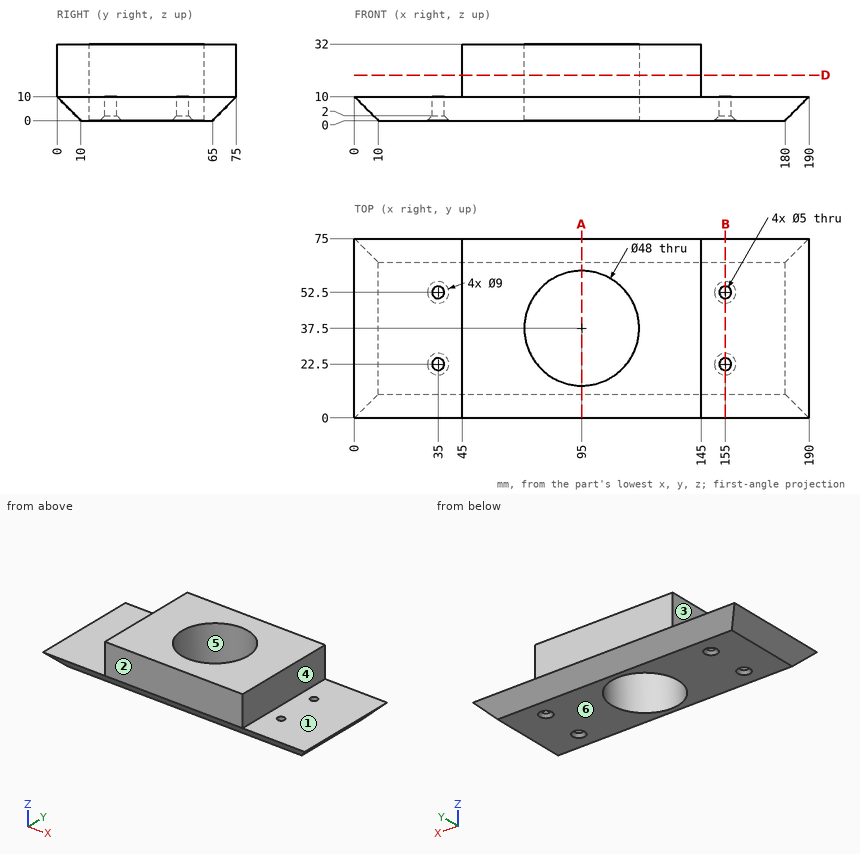
Could you check a few things on this drawing? It's one solid part, dimensions in mm from its lowest x, y, z. A direction names the side the tool comes from. Give positions to 0.01 mm unless a question says otherwise; leave off trailing zeros. Order: outer loops, then holes, each group sorted by start corner. A loop starts at its lowest first (then second) coordinate and runs counter-clockwise, first axis right, second up. Notation, with made-up numbers: (1, 31.5) - (5, 31.5) arc R19 cw to (5, 66.5) - close; hole circle Ø5 at (-15, -20.75). An arc over 180 degrees is marked (long way). One line per question, with ' | ' between items. Start each with the question number.
Item 1: Thinking about a two-plate mould opening in X: for the marked faces 4, 5 and 6, which applies, pulls with the +X half, pulls with the -X half, needs draft (parallel to the pull), parting line crosses it, or undercut?
Item 2: I need wall thicknesses on probe 1 along Y at (x, z) = (96, 11.5); probe 2 along Y at (x, z) = (35, 6); probe 3 along X at (y, z) = (52, 4). Which ranges of each line are inside material? Lowest first, please. Write a range as [from, to].
Item 3: I'm going to push flat-ended pins straight in: pin 1 Ø8 at (x, y) = (44.5, 19.5) entering from -Z; pin 2 Ø6.5 at (y, z) = (49.5, 17.5) entering from -X; pin 3 Ø22.5 at (x, y) = (14.5, 27) entering from +Z; pin 4 Ø5 at (y, z) = (32, 23) entering from +X. Where does each tip first touch, or does it pass through?
Item 4: I want a section at D-D on z = 19. Write out the boundary of the cut face in (x, y), then the cut area to 3 significant figures.
Item 5: For the marked faces 1, 2 and 3, which set-ups out of +Z, -Z, +X, -X, +Y, -Y let a thin tool reach every point of the face, with its end or its side?
Item 6: I want a section at B-B on x = 155. Give the number of separate pieces and of enclosed holes in the cut face, then the cut area to 3 significant figures.
Item 7: I want a section at A-A on x = 95. Write out the boundary of the cut face in (y, z), then the cut area to 3 significant figures.
Verdict:
1) face 4: pulls with the +X half | face 5: undercut | face 6: needs draft
2) probe 1: [0, 13.52], [61.48, 75] | probe 2: [4, 20], [25, 50], [55, 71] | probe 3: [6, 32.55], [37.45, 75.88], [114.12, 152.55], [157.45, 184]
3) pin 1: z = 0 | pin 2: x = 45 | pin 3: z = 10 | pin 4: x = 145
4) outline: (45, 0) - (145, 0) - (145, 75) - (45, 75) - close; hole circle Ø48 at (95, 37.5) | area: 5,690 mm^2
5) face 1: +Z, +X, +Y, -Y | face 2: +Z, -Z, +X, -X, -Y | face 3: +Z, -X, +Y, -Y
6) separate pieces: 3 | enclosed holes: 0 | area: 542 mm^2
7) outline: (0, 10) - (10, 0) - (13.5, 0) - (13.5, 32) - (0, 32) - close; (61.5, 0) - (65, 0) - (75, 10) - (75, 32) - (61.5, 32) - close | area: 764 mm^2
